Here's the drawing with two shaded views (mm, measured from the low corner). I have some questions. A direction names the side the tool comes from. Coordinates: 2 decimals unless noted, no trailing zeros. Order: outer loops, then holes, each group sorted by start corner. A loop starts at its lowest first (then second) coordinate and runs counter-clockwise, first axis right, second up. Notation, with made-up numbers: (19.5, 7.5) -> (60.5, 7.5) arc R13 cw to (60.5, 13.5) -> close; hole circle Ø2 at (38.5, 55). An arc over 180 degrees is marked (long way). Answer in a Markdown table with one row per item. Add a question column.
1. We'd pull the mould along X, two halves only. Please class the marked faces 1 and 2: pulls with the +X half, pulls with the -X half, needs draft (parallel to the pull), parting line crosses it, or undercut.
2. Imagine slicing it at B-B on x = 9. Write out the boundary of the cut face in (y, z).
3. Imagine slicing it at C-C on y = 35. Write out the boundary of the cut face in (x, z).
4. Imagine slicing it at A-A on z = 9. Write out the boundary of the cut face in (x, y).
5. On a 3-axis mill with a long thin cutter (end or side, diameter ignored), from which of +Z, -Z, +X, -X, +Y, -Y can I reach the whole of each face in a straight line? I mean the marked faces 3 and 4. Say none if no direction works.
6. If I drill on line 1 along X through (y, z) = (36.5, 9); line 2 along X through (y, z) = (58.5, 2.75), over which ranges is the centre line in solid material (lowest first)? Write a range as [from, to].
7. Will these pins go through, and if not, where does the flat tip stop? pin 1 (4 mm diameter, centred on y = 23.5, z = 12, fed in from -X); pin 2 (2 mm diameter, centred on x = 7.5, y = 62.5, fed in from -Z); pin 3 (2 mm diameter, centred on x = 11.5, y = 34.5, fed in from +Z).
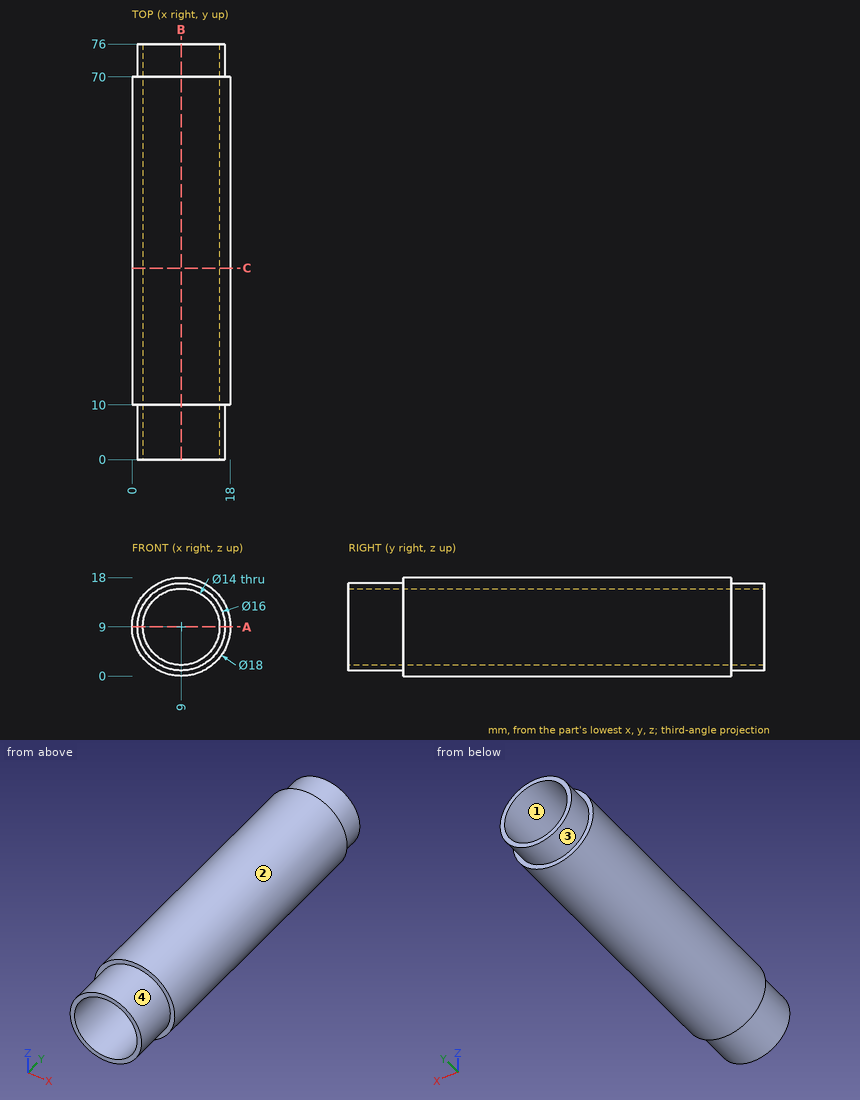
Answers follow:
| question | item | result |
|---|---|---|
| 1 | face 1 | undercut |
| 1 | face 2 | parting line crosses it |
| 2 | outline | (0, 1) -> (10, 1) -> (10, 0) -> (70, 0) -> (70, 1) -> (76, 1) -> (76, 2) -> (0, 2) -> close; (0, 16) -> (76, 16) -> (76, 17) -> (70, 17) -> (70, 18) -> (10, 18) -> (10, 17) -> (0, 17) -> close |
| 3 | outline | circle Ø18 at (9, 9); hole circle Ø14 at (9, 9) |
| 4 | outline | (0, 10) -> (1, 10) -> (1, 0) -> (2, 0) -> (2, 76) -> (1, 76) -> (1, 70) -> (0, 70) -> close; (16, 0) -> (17, 0) -> (17, 10) -> (18, 10) -> (18, 70) -> (17, 70) -> (17, 76) -> (16, 76) -> close |
| 5 | face 3 | +Y |
| 5 | face 4 | -Y |
| 6 | line 1 | x = [0, 2], [16, 18] |
| 6 | line 2 | x = [2.52, 5.85], [12.15, 15.48] |
| 7 | pin 1 | stops at x = 0.06 |
| 7 | pin 2 | stops at z = 0.01 |
| 7 | pin 3 | stops at z = 17.87 |
